Part model, mm, in its own coordinate system. A direction names the side the tool comes from. Round coordinates to 2 decimals unless told otherwise and drop trailing zeros. Write each loop counter-clockwise with the first axis right and the second up, starting at its lowest first coordinate (ties: lowest second). Pieces come first, ordered by that corner, then holes. Notation, with made-up numbers: M 85,6.25 L 96,6.25 A19 ccw 96,41.25 Z; hole C -10.75,60 d9. An arc over 180 degrees is marked long. Use a Markdown table: item, result. Add a question column.
1) Drop flat-ended pins along their axis: P1, Ø5, axis at y = 423, z = 9.5, coming from the -X side; P2, Ø4, axis at x = 62, z = -20, coming from the +Y side; P3, Ø1, axis at x = -12, z = -1.5, coming from the -Y side. Give the stop position or say it passes through.
2) Two-plate mould, pull along X, no slides. Class faces 4 (the face through (-1, 386, -25.4)), 5 (the face through (25.756, 755.993, 0.356)), 6 (the face through (101.6, 50, 0)): released by +X, released by -X, zero draft, split by the parting line, or undercut.
3) Slice it at A-A on z = 15. Write the cut outline in (x, y).
4) Which spindle directions (+Z, -Z, +X, -X, +Y, -Y) get a long thin tool onto all of the face, cutting with end or side? Do faces 1 (the face through (-76.2, 38, 0)), 2 (the face through (-25.044, 755.815, 0.356)), 3 (the face through (50.8, 427, 0)). Say none if no direction does.
5) Wall check: probe 1 along X at (y, z) = (64.5, 3.5); probe 2 along X at (y, z) = (589, -2); probe 3 along Y at (x, z) = (64.5, 4.5). Give the ranges that are in metal, low to high.
6) Slice it at C-C on y = 552.5. Write the cut outline in (x, z), plus the area to 3 significant figures.
7) Slice it at B-B on x = 84.5. Write the cut outline in (y, z), plus the area to 3 significant figures.
```python
from build123d import *

# Parameters (mm, degrees)
BOSS_EXTRUDE1_DEPTH = 25.4


with BuildPart() as part:
    # Sketch1 → Boss-Extrude1 (new body, symmetric)
    with BuildSketch(Plane.XY):
        Polygon((0, 749.554), (-50.8, 762.254), (-50.8, 101.6), (-101.6, 101.6), (-101.6, 0), (-76.2, 0), (-76.2, 76.2), (0, 76.2), (76.2, 76.2), (76.2, 0), (101.6, 0), (101.6, 101.6), (50.8, 101.6), (50.8, 762.254), align=None)
    extrude(amount=BOSS_EXTRUDE1_DEPTH, both=True)


solid = part.part
```
Entries:
| question | item | result |
|---|---|---|
| 1 | P1 | stops at x = -50.8 |
| 1 | P2 | stops at y = 101.6 |
| 1 | P3 | stops at y = 76.2 |
| 2 | face 4 | zero draft |
| 2 | face 5 | undercut |
| 2 | face 6 | released by +X |
| 3 | outline | M -101.6,0 L -76.2,0 L -76.2,76.2 L 76.2,76.2 L 76.2,0 L 101.6,0 L 101.6,101.6 L 50.8,101.6 L 50.8,762.25 L 0,749.55 L -50.8,762.25 L -50.8,101.6 L -101.6,101.6 Z |
| 4 | face 1 | +Z, -Z, -Y |
| 4 | face 2 | +Z, -Z, +Y |
| 4 | face 3 | +Z, -Z, +X, +Y |
| 5 | probe 1 | x = -101.6 to -76.2, 76.2 to 101.6 |
| 5 | probe 2 | x = -50.8 to 50.8 |
| 5 | probe 3 | y = 76.2 to 101.6 |
| 6 | outline | M -50.8,-25.4 L 50.8,-25.4 L 50.8,25.4 L -50.8,25.4 Z |
| 6 | area | 5,160 mm^2 |
| 7 | outline | M 0,-25.4 L 101.6,-25.4 L 101.6,25.4 L 0,25.4 Z |
| 7 | area | 5,160 mm^2 |
